The figure shows three views and two pictorial views of one solid part (mm, origin at its lowest corner). Answer the questions. A direction names the side the tool comes from. Coordinates: 2 decimals unless noted, no trailing zeros. Write each loop counter-clockwise with the first axis right and the second up, starting at its lowest first coordinate (ties: lowest second). Pieces come first, ordered by that corner, then holes.
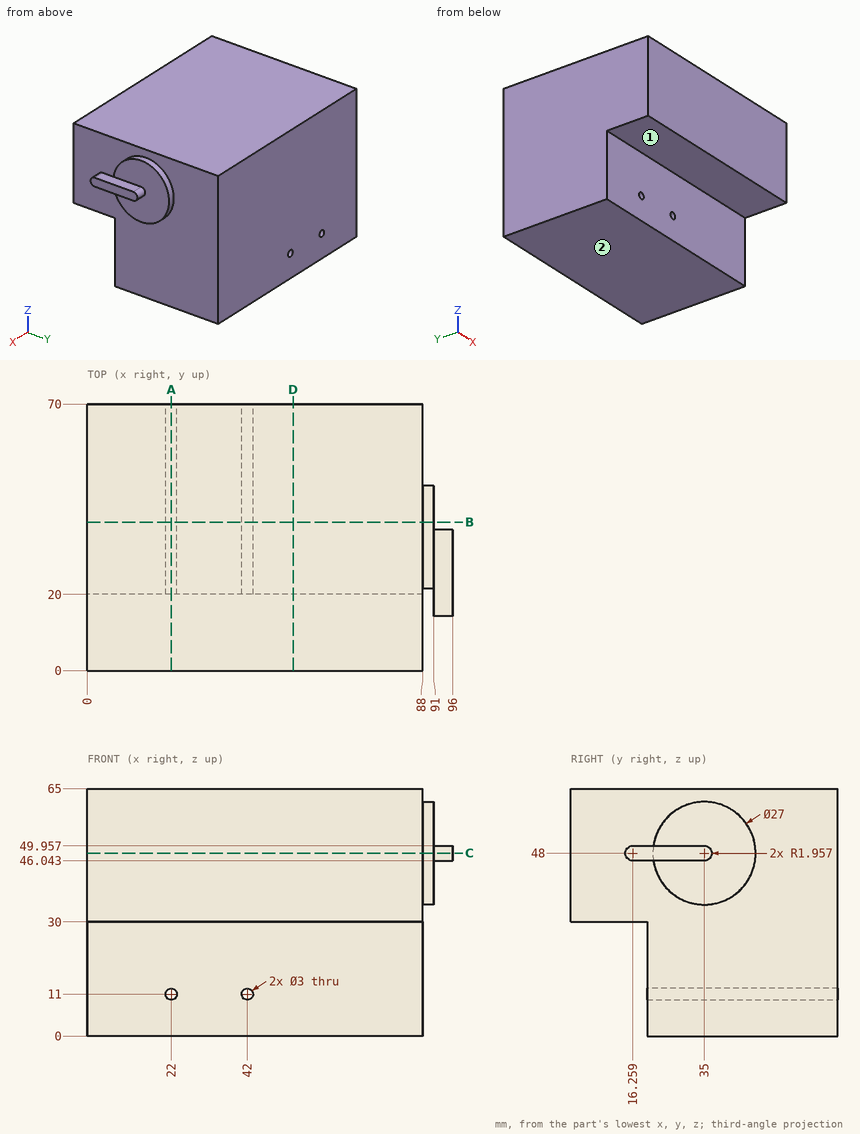
Q1. Which of the six approach directions +Z, -Z, +X, -X, +Y, -Y give full straight-line access (tool end or side, diameter ignored) to the marked faces 1 and 2?
Answers below:
face 1: -Z, +X, -X, -Y
face 2: -Z, +X, -X, +Y, -Y
Q2. Find the intervals of material crossed by probe 1 along X at (y, z) = (41, 11); probe 2 along Y at (x, z) = (72, 8.5); probe 3 along X at (y, z) = (42, 7), in increasing order.
Answers below:
probe 1: x = 0 to 20.5, 23.5 to 40.5, 43.5 to 88
probe 2: y = 20 to 70
probe 3: x = 0 to 88
Q3. Given pin 1 (9 mm diameter, centred on x = 30.5, z = 19, fed in from -Y); pin 2 (2 mm diameter, centred on y = 41.5, z = 34.5, fed in from +X); pin 3 (2.5 mm diameter, centred on x = 94.5, y = 25.5, fed in from +Z), each flat-ended and moving along its own axis, determine where each tip first touches the part or whether it passes through.
Answers below:
pin 1: stops at y = 20
pin 2: stops at x = 88
pin 3: stops at z = 49.96
Q4. The part is cut by section D-D, the plane x = 54. Write down the section's boundary in (y, z).
Answers below:
outline: (0, 30) - (20, 30) - (20, 0) - (70, 0) - (70, 65) - (0, 65) - close
Q5. The part is cut by section B-B, the plane y = 39. Write down the section's boundary in (x, z).
Answers below:
outline: (0, 0) - (88, 0) - (88, 35.11) - (91, 35.11) - (91, 60.89) - (88, 60.89) - (88, 65) - (0, 65) - close; hole circle Ø3 at (22, 11); hole circle Ø3 at (42, 11)
Q6. The part is cut by section C-C, the plane z = 48. Write down the section's boundary in (x, y), then the cut area to 3 significant figures.
Answers below:
outline: (0, 0) - (88, 0) - (88, 21.5) - (91, 21.5) - (91, 14.3) - (96, 14.3) - (96, 36.96) - (91, 36.96) - (91, 48.5) - (88, 48.5) - (88, 70) - (0, 70) - close
area: 6,350 mm2
Q7. The part is cut by section A-A, the plane x = 22. Write down the section's boundary in (y, z).
Answers below:
outline: (0, 30) - (20, 30) - (20, 12.5) - (70, 12.5) - (70, 65) - (0, 65) - close; (20, 0) - (70, 0) - (70, 9.5) - (20, 9.5) - close
